```python
from build123d import *

# Parameters (mm, degrees)
F1_DEPTH = 25.4
F0_W     = 30.6482749184
F0_H     = 19.05
F0_H_2   = 4.7752
F2_DEPTH = 12.7
F3_DEPTH = 25.4


with BuildPart() as f1:
    # F0 (on Front) → F1 (new body)
    with BuildSketch(Plane.XZ):
        Polygon((-44.7792303854, -9.525), (37.7707696146, -9.525), (37.7707696146, 9.525), (18.7207696146, 9.525), (-44.7792303854, 9.525), align=None)
    extrude(amount=-F1_DEPTH)

    # F0 (on Front) → F2 (join, symmetric)
    with BuildSketch(Plane.XZ):
        Polygon((-44.7792303854, -9.525), (37.7707696146, -9.525), (37.7707696146, 9.525), (18.7207696146, 9.525), (-44.7792303854, 9.525), align=None)
        with BuildLine():
            Line((18.7207696146, 9.525), (37.7707696146, 9.525))
            Line((37.7707696146, 9.525), (37.7707696146, 27.1368854333))
            ThreePointArc((37.7707696146, 27.1368854333), (43.1811641643, 39.0745425639), (55.7244902785, 42.8752))
            Line((55.7244902785, 42.8752), (56.8207696146, 42.8752))
            Line((56.8207696146, 42.8752), (56.8207696146, 61.9252))
            Line((56.8207696146, 61.9252), (56.7326441838, 61.9252))
            ThreePointArc((56.7326441838, 61.9252), (30.0666842775, 52.9008594991), (18.7207696146, 27.1368854333))
            Line((18.7207696146, 27.1368854333), (18.7207696146, 9.525))
        make_face()
        with BuildLine():
            add(Edge.make_bspline(
                [(-44.7792303854, 9.525), (-50.61746484, 47.9471649566), (18.7515171766, 66.2469923459), (56.7326441838, 61.9252)],
                knots=[0, 0, 0, 0, 114.2385295712, 114.2385295712, 114.2385295712, 114.2385295712], degree=3))
            Line((-44.7792303854, 9.525), (18.7207696146, 9.525))
            Line((18.7207696146, 9.525), (18.7207696146, 27.1368854333))
            ThreePointArc((18.7207696146, 27.1368854333), (30.0666842775, 52.9008594991), (56.7326441838, 61.9252))
        make_face()
        with Locations((72.1449070738, 52.4002)):
            Rectangle(F0_W, F0_H)
        Polygon((56.8207696146, 66.675), (56.8207696146, 61.9252), (87.469044533, 61.9252), (87.469044533, 42.8752), (87.469044533, 38.1), (107.6207696146, 38.1), (107.6207696146, 66.675), align=None)
        with Locations((72.1449070738, 40.4876)):
            Rectangle(F0_W, F0_H_2)
    extrude(amount=F2_DEPTH, both=True)

    # F0 (on Front) → F3 (join)
    with BuildSketch(Plane.XZ):
        Polygon((-44.7792303854, -9.525), (37.7707696146, -9.525), (37.7707696146, 9.525), (18.7207696146, 9.525), (-44.7792303854, 9.525), align=None)
        with BuildLine():
            Line((18.7207696146, 9.525), (37.7707696146, 9.525))
            Line((37.7707696146, 9.525), (37.7707696146, 27.1368854333))
            ThreePointArc((37.7707696146, 27.1368854333), (43.1811641643, 39.0745425639), (55.7244902785, 42.8752))
            Line((55.7244902785, 42.8752), (56.8207696146, 42.8752))
            Line((56.8207696146, 42.8752), (56.8207696146, 61.9252))
            Line((56.8207696146, 61.9252), (56.7326441838, 61.9252))
            ThreePointArc((56.7326441838, 61.9252), (30.0666842775, 52.9008594991), (18.7207696146, 27.1368854333))
            Line((18.7207696146, 27.1368854333), (18.7207696146, 9.525))
        make_face()
        with BuildLine():
            add(Edge.make_bspline(
                [(-44.7792303854, 9.525), (-50.61746484, 47.9471649566), (18.7515171766, 66.2469923459), (56.7326441838, 61.9252)],
                knots=[0, 0, 0, 0, 114.2385295712, 114.2385295712, 114.2385295712, 114.2385295712], degree=3))
            Line((-44.7792303854, 9.525), (18.7207696146, 9.525))
            Line((18.7207696146, 9.525), (18.7207696146, 27.1368854333))
            ThreePointArc((18.7207696146, 27.1368854333), (30.0666842775, 52.9008594991), (56.7326441838, 61.9252))
        make_face()
        with Locations((72.1449070738, 52.4002)):
            Rectangle(F0_W, F0_H)
        Polygon((56.8207696146, 66.675), (56.8207696146, 61.9252), (87.469044533, 61.9252), (87.469044533, 42.8752), (87.469044533, 38.1), (107.6207696146, 38.1), (107.6207696146, 66.675), align=None)
        with Locations((72.1449070738, 40.4876)):
            Rectangle(F0_W, F0_H_2)
    extrude(amount=F3_DEPTH)


solid = f1.part
```
Source: CAD feature listing. Evaluate the final solid. Frame: model axes, mm. A direction names the side the tool comes from. Give positions to 0.01 mm unless a question says otherwise; leave off trailing zeros. Loops run counter-clockwise (first coordinate to the right, second up) from the corner with the lowest first, then second, coordinate; pieces in that order, holes last. Notation, with made-up numbers: (3, 30) - (61, 30) arc R16 ccw to (61, 40) - close; hole circle Ø2 at (13, 63.5). An arc over 180 degrees is marked (long way). Use CSV: the item, a comma, the result in double quotes. Start each with the question number.
1. Section B-B (x = 85.5). Output: boundary loops of the cut face in (y, z) (3 decimals).
2. Reachability of faces 1 (the flat face through (-44.779, 0, 0)), 2 (the flat face through (56.821, -6, 40)), 3 (the flat face through (-3, 19, 9.525)), 4 (the flat face through (10, -25.4, 29)), 5 (the flat face through (37.771, 0, 9)) from +Z, -Z, +X, -X, +Y, -Y: full face, straight path, thin tool, end or side. Return the list, or none.
3. Ray query, L1, parallel to X at y = -19, z = -2; L2, parallel to Z at x = 96, y = 7 (3 decimals); L3, parallel to Y at x = -23, z = 41.5. Return the intervals inside material, ascending.
4. Section A-A (y = 20.5). Output: boundary loops of the cut face in (x, z) (3 decimals), then the cut area to 3 significant figures.
5. Pin query (flat end, axial travel): pin 1 (17 mm diameter, centred on x = 57, z = 37, fed in from +Y); pin 2 (8 mm diameter, centred on y = -10, z = 42, fed in from -X); pin 3 (1.5 mm diameter, centred on y = 14.5, z = 9.5, fed in from -X). Return the tip coordinate at first contact, or that it passes through.
Response:
1,outline,"(-25.4, 38.1) - (12.7, 38.1) - (12.7, 66.675) - (-25.4, 66.675) - close"
2,face 1,"-Z, -X, +Y, -Y"
2,face 2,"-Z, +Y, -Y"
2,face 3,"+Z, +X, -X, +Y"
2,face 4,"+Z, -Z, +X, -X, -Y"
2,face 5,"-Z, +X, +Y, -Y"
3,L1,"-44.78 to 37.77"
3,L2,"38.1 to 66.675"
3,L3,"-25.4 to 12.7"
4,outline,"(-44.779, -9.525) - (37.771, -9.525) - (37.771, 9.525) - (-44.779, 9.525) - close"
4,area,"1,570 mm²"
5,pin 1,"y = 12.7"
5,pin 2,"x = -33.28"
5,pin 3,"x = -44.78"
